Autodesk Inventor part; units mm, degrees
ref_plane "YZ Plane" through (0, 0, 0) normal (1, 0, 0) x (0, 1, 0)
ref_plane "XZ Plane" through (0, 0, 0) normal (0, 1, 0) x (-1, 0, 0)
ref_plane "XY Plane" through (0, 0, 0) normal (0, 0, 1) x (1, 0, 0)
sketch "Sketch1" plane through (0, 0, 0) normal (0, 0, 1) x (1, 0, 0)
  circle A0 centre (0, 0) radius 25
  line L0 (0, 0) -> (20, 0) construction
  dimension "d0" = 50
  dimension "d1" = 20
extrude "Extrusion1" add sketch "Sketch1" along normal blind 16
sketch "Sketch2" plane through (0, 0, 16) normal (0, 0, 1) x (1, 0, 0)
  circle A0 centre (0, 0) radius 25
  point P0 (-14.1421, 14.1421)
  point P1 (-14.1421, -14.1421)
  point P2 (14.1421, -14.1421)
  point P3 (14.1421, 14.1421)
  dimension "d18" = 360
hole "Hole1" at (-14.1421, 14.1421, 16) at (-14.1421, -14.1421, 16) at (14.1421, -14.1421, 16) at (14.1421, 14.1421, 16) direction (0, 0, -1) diameter 6.5 end through all
sketch "Sketch11" plane through (0, 0, 16) normal (0, 0, 1) x (1, 0, 0)
  line L0 (0, 0) -> (20, 0)
  dimension "d68" = 20
hole "Hole4" at (20, 0, 16) direction (0, 0, -1) diameter 6.5 end through all
sketch "Sketch12" plane through (0, 0, 16) normal (0, 0, 1) x (1, 0, 0)
  circle A0 centre (0, 0) radius 10.5
  dimension "d76" = 21
extrude "Extrusion7" add sketch "Sketch12" along normal blind 25
properties part number "BaseImpresion" material "PVC-Piping"
Read the model definition and answer for the solid it produces. Units are mm, in the model's axes. A direction names the side the tool comes from. Give positions to 0.01 mm unless a question says otherwise; leave off trailing zeros. Order: outer loops, then holes, each group sorted by start corner. A loop starts at its lowest first (then second) coordinate and runs counter-clockwise, first axis right, second up. Notation, with made-up numbers: (73.25, 71) -> (116.25, 71) arc R25 cw to (116.25, 103) -> close; hole circle Ø9 at (17, 71). An arc over 180 degrees is marked (long way). Write item = value, one per line.
1. For faces 1 (the face through (16.778, 0.423, 7.888)), 2 (the face through (0, -11, 16)), determine the directions among +Z, -Z, +X, -X, +Y, -Y from which every point of the face is accessible in a straight line to the end or side of a thin tool.
Numbers:
face_1 = +Z, -Z
face_2 = +Z
2. Given pin 1 (3 mm diameter, centred on y = -4.5, z = 25.5, fed in from -X); pin 2 (3 mm diameter, centred on x = -16, y = -1.5, fed in from +Z); pin 3 (8 mm diameter, centred on y = -17, z = 6.5, fed in from +X), each flat-ended and moving along its own axis, determine where each tip first touches the part or whether it passes through.
Numbers:
pin_1 = -10.06
pin_2 = 16
pin_3 = 21.35
3. The mould has two halves that part along X. Classify faces 3 (the face through (10, -3.2, 28.3)), 4 (the face through (14, 17.39, 7.89)), 5 (the face through (0, 0, 0)): +X half, -X half, draft (parallel to the pull), parting line (faces both ways), or undercut.
Numbers:
face_3 = parting line
face_4 = undercut
face_5 = draft
4. A cutting plane is placed at D-D, the plane z = 8.5. Write down the section's boundary in (x, y), and give its area (3 significant figures).
Numbers:
outline = circle Ø50 at (0, 0); hole circle Ø6.5 at (-14.14, -14.14); hole circle Ø6.5 at (-14.14, 14.14); hole circle Ø6.5 at (14.14, -14.14); hole circle Ø6.5 at (14.14, 14.14); hole circle Ø6.5 at (20, 0)
area = 1,800 mm²
5. Straight lines are drawn through the part: line 1 along Y through (x, z) = (-12, 14.5); line 2 along X through (y, z) = (13.5, 14); line 3 along Z through (x, y) = (9, 10). For each, find the intervals that lie inside material, in ascending order.
Numbers:
line_1 = -21.93 to -16.59, -11.7 to 11.7, 16.59 to 21.93
line_2 = -21.04 to -17.33, -10.96 to 10.96, 17.33 to 21.04
line_3 = 0 to 16
6. A cutting plane is placed at A-A, the plane y = 0. Write down the section's boundary in (x, z).
Numbers:
outline = (-25, 0) -> (16.75, 0) -> (16.75, 16) -> (10.5, 16) -> (10.5, 41) -> (-10.5, 41) -> (-10.5, 16) -> (-25, 16) -> close; (23.25, 0) -> (25, 0) -> (25, 16) -> (23.25, 16) -> close
7. A cutting plane is placed at C-C, the plane x = 0. Write down the section's boundary in (y, z).
Numbers:
outline = (-25, 0) -> (25, 0) -> (25, 16) -> (10.5, 16) -> (10.5, 41) -> (-10.5, 41) -> (-10.5, 16) -> (-25, 16) -> close
8. A cutting plane is placed at B-B, the plane x = 20. Write down the section's boundary in (y, z).
Numbers:
outline = (-15, 0) -> (-3.25, 0) -> (-3.25, 16) -> (-15, 16) -> close; (3.25, 0) -> (15, 0) -> (15, 16) -> (3.25, 16) -> close
